Design review of the part built by this model. Coordinates are the model's own, in mm. A direction names the side the tool comes from. Give positions to 0.01 mm unless a question says otherwise; leave off trailing zeros. Order: outer loops, then holes, each group sorted by start corner. A loop starts at its lowest first (then second) coordinate and runs counter-clockwise, first axis right, second up. Notation, with made-up numbers: (63.5, -28.5) -> (86.5, -28.5) arc R26 ccw to (86.5, 2.5) -> close; hole circle Ø2 at (76, 12.5). An arc over 180 degrees is marked (long way). One line per item, written item: value.
from build123d import *

# Parameters (mm, degrees)
SKETCH1_R                   = 62
BOSS_EXTRUDE1_DEPTH         = 15
SKETCH2_R                   = 2
CUT_EXTRUDE1_DEPTH          = 15
CIRPATTERN1_COUNT           = 2
CIRPATTERN1_ANGLE           = 60
CIRPATTERN2_COUNT           = 2
CIRPATTERN2_COPY_1_SKETCH_R = 2
CIRPATTERN2_COPY_1_DEPTH    = 15
SKETCH3_R                   = 6.1
CUT_EXTRUDE2_DEPTH          = 15
SKETCH4_R                   = 2.5
CUT_EXTRUDE4_DEPTH          = 10
CIRPATTERN5_COUNT           = 5


with BuildPart() as part:
    # Sketch1 → Boss-Extrude1 (new body)
    with BuildSketch(Plane.XY):
        Circle(SKETCH1_R)
    extrude(amount=BOSS_EXTRUDE1_DEPTH)

    # Sketch2 → Cut-Extrude1 (cut)
    with BuildSketch(Plane.XY.offset(15)):
        with Locations((0, 49.5)):
            Circle(SKETCH2_R)
    cut_extrude1 = extrude(amount=-CUT_EXTRUDE1_DEPTH, mode=Mode.SUBTRACT)

    # CirPattern1: Cut-Extrude1 ×2 about axis
    cirpattern1_axis = Axis((0, 0, 15), (0, 0, -1))
    for i in range(1, CIRPATTERN1_COUNT):
        add(cut_extrude1.rotate(cirpattern1_axis, i * CIRPATTERN1_ANGLE / (CIRPATTERN1_COUNT - 1)), mode=Mode.SUBTRACT)

    # CirPattern2: Cut-Extrude1 ×2 about axis
    cirpattern2_axis = Axis((0, 0, 0), (0, 0, 1))
    for i in range(1, CIRPATTERN2_COUNT):
        add(cut_extrude1.rotate(cirpattern2_axis, i * 360 / CIRPATTERN2_COUNT), mode=Mode.SUBTRACT)

    # CirPattern2 copy 1 sketch → CirPattern2 copy 1 (cut)
    with BuildSketch(Plane(origin=(0, 0, 15), x_dir=(-0.49999999999999767, 0.86602540378444, 0), z_dir=(0, 0, 1))):
        with Locations((0, 49.5)):
            Circle(CIRPATTERN2_COPY_1_SKETCH_R)
    extrude(amount=-CIRPATTERN2_COPY_1_DEPTH, mode=Mode.SUBTRACT)

    # Sketch3 → Cut-Extrude2 (cut)
    with BuildSketch(Plane.XY.offset(15)):
        Circle(SKETCH3_R)
    extrude(amount=-CUT_EXTRUDE2_DEPTH, mode=Mode.SUBTRACT)

    # Sketch4 → Cut-Extrude4 (cut)
    with BuildSketch(Plane(origin=(51.997575213, 33.767620171, 0), x_dir=(0, 0, -1), z_dir=(-0.8386705679454236, -0.544639035015028, 0))):
        with Locations(Location((-7.5, 0, 0), (0, 0, 270))):
            Circle(SKETCH4_R)
    cut_extrude4 = extrude(amount=CUT_EXTRUDE4_DEPTH, mode=Mode.SUBTRACT)

    # CirPattern5: Cut-Extrude4 ×5 about axis
    cirpattern5_axis = Axis((0, 0, 0), (0, 0, 1))
    for i in range(1, CIRPATTERN5_COUNT):
        add(cut_extrude4.rotate(cirpattern5_axis, i * 360 / CIRPATTERN5_COUNT), mode=Mode.SUBTRACT)


solid = part.part
Item 1: Add section D-D on y = 11. Give the boundary of the cut face in (x, z).
Returned:
outline: (-61.02, 0) -> (61.02, 0) -> (61.02, 15) -> (-61.02, 15) -> close
Item 2: Add section A-A on y = 24.75. Give the boundary of the cut face in (x, z).
Returned:
outline: (-56.85, 0) -> (40.87, 0) -> (40.87, 15) -> (-56.85, 15) -> close; (44.87, 0) -> (56.85, 0) -> (56.85, 15) -> (44.87, 15) -> close
Item 3: Draft analysis for pull direction Z (two halves, no side actions). For faces 3 (the cylindrical face through (0.923, 47.726, 7.605)), 4 (the flat face through (40.39, -32.75, 7.46)), 5 (the flat face through (-1, -13, 0)), state which applies: pulls with the +Z half, pulls with the -Z half, needs draft (parallel to the pull), parting line crosses it, or undercut.
Returned:
face 3: needs draft
face 4: undercut
face 5: pulls with the -Z half
Item 4: Clearance check with flat-ended pins moving along their axes: P1, Ø3, axis at x = -20.5, z = 7, coming from the -Y side; P2, Ø1.5, axis at x = 15, z = 3.5, coming from the +Y side; P3, Ø6, axis at y = 40, z = 6.5, coming from the +X side. State where each tip first meets the part, or that it passes through.
Returned:
P1: y = -59.02
P2: y = 60.34
P3: x = 49.75
Item 5: Machinability: for faces 1 (the flat face through (-1, -13, 15)), 2 (the flat face through (-18.668, -48.534, 7.465)), which of the approach directions +Z, -Z, +X, -X, +Y, -Y give a long, thin tool a straight path to every point of the face, cutting with its end or side? Answer none if there is none.
Returned:
face 1: +Z, +X, -X, +Y, -Y
face 2: none
Item 6: Add section C-C on x = 17.5. Give the boundary of the cut face in (y, z).
Returned:
outline: (-59.48, 0) -> (59.48, 0) -> (59.48, 15) -> (-59.48, 15) -> close
Item 7: Add section B-B on z = 3. Give the boundary of the cut face in (x, y), plus the area to 3 significant figures.
Returned:
outline: circle Ø124 at (0, 0); hole circle Ø4 at (-42.87, -24.75); hole circle Ø12.2 at (0, 0); hole circle Ø4 at (0, -49.5); hole circle Ø4 at (0, 49.5); hole circle Ø4 at (42.87, 24.75)
area: 11,900 mm²
Item 8: To check wall thickness, follow line 1 along Y through (x, z) = (0, 4.75); line 2 along Y through (x, z) = (-3, 1.5); line 3 along X through (y, z) = (-5, 9.25). State the ranges of each line that lie inside material, in increasing order. Write a range as from..to.
Returned:
line 1: -62..-51.5, -47.5..-6.1, 6.1..47.5, 51.5..62
line 2: -61.93..-5.31, 5.31..61.93
line 3: -61.8..-3.49, 3.49..61.8
